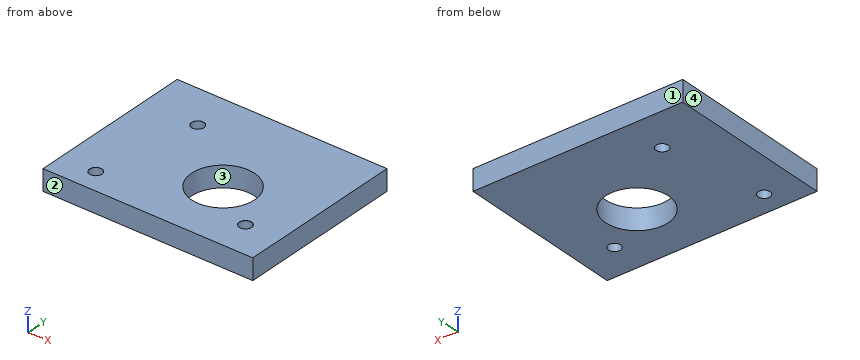
```python
from build123d import *

# Parameters (mm, degrees)
SKETCH1_W                        = 50
SKETCH1_H                        = 40
BOSS_EXTRUDE1_DEPTH              = 2.5
M2_5_CLEARANCE_HOLE2_D           = 2.9
M2_5_CLEARANCE_HOLE2_CSINK_D     = 2.95
M2_5_CLEARANCE_HOLE2_CSINK_ANGLE = 90
SKETCH4_R                        = 7.5
CUT_EXTRUDE1_DEPTH               = 6


with BuildPart() as part:
    # Sketch1 → Boss-Extrude1 (new body, symmetric)
    with BuildSketch(Plane.XY):
        with Locations((16.688846575, 14.654391813)):
            Rectangle(SKETCH1_W, SKETCH1_H)
    extrude(amount=BOSS_EXTRUDE1_DEPTH, both=True)

    # M2.5 Clearance Hole2 (through all)
    with Locations(Plane.XY.offset(2.5)):
        with Locations((4.655068225, 24.562783633), (33.37769315, 2.86), (0, 0)):
            CounterSinkHole(M2_5_CLEARANCE_HOLE2_D / 2, M2_5_CLEARANCE_HOLE2_CSINK_D / 2, counter_sink_angle=M2_5_CLEARANCE_HOLE2_CSINK_ANGLE)

    # Sketch4 → Cut-Extrude1 (cut, through all)
    with BuildSketch(Plane.XY.offset(2.5)):
        with Locations((21.775361697, 10.694915753)):
            Circle(SKETCH4_R)
    extrude(amount=-CUT_EXTRUDE1_DEPTH, mode=Mode.SUBTRACT)


solid = part.part
```
Here's how the part is built. I have some questions about the finished solid (model axes, mm). Face numbers are marked on the shaded views. Round coordinates to 2 decimals unless told otherwise and drop trailing zeros. Write each loop counter-clockwise with the first axis right and the second up, starting at its lowest first coordinate (ties: lowest second). Pieces come first, ordered by that corner, then holes.
Q1. Will this pin go through, and if not, where does the flat tip stop? P1, Ø9, axis at x = 21.78, y = 10.69, coming from the +Z side.
Q2. If we section it at C-C on z = 0.05: Write out the boundary of the cut face in (x, y).
Q3. If we section it at B-B on x = 0: Write out the boundary of the cut face in (y, z) (3 decimals).
Q4. Please list where these lines run through material, in increasing order: probe 1 along X at (y, z) = (2.86, 1.2); probe 2 along X at (y, z) = (0, 1.1); probe 3 along Y at (x, z) = (21.5, 0.45).
Q5. If we mould it in two halves opening along Y, with no side actions, what happens to the marked faces 1, 2, 3 and 4? For each: +Y half, -Y half, draft (parallel to the pull), parting line (faces both ways), or undercut.
Q6. If we section it at D-D on y = 16: Write out the boundary of the cut face in (x, z).
Q7. If we section it at A-A on y = 0: Write out the boundary of the cut face in (x, z) (3 decimals), plus the area to 4 significant figures.
Answer below:
1. P1: passes through
2. outline: (-8.31, -5.35) - (41.69, -5.35) - (41.69, 34.65) - (-8.31, 34.65) - close; hole circle Ø2.9 at (0, 0); hole circle Ø2.9 at (4.66, 24.56); hole circle Ø15 at (21.78, 10.69); hole circle Ø2.9 at (33.38, 2.86)
3. outline: (-5.346, -2.5) - (-1.45, -2.5) - (-1.45, 2.475) - (-1.475, 2.5) - (-5.346, 2.5) - close; (1.45, -2.5) - (34.654, -2.5) - (34.654, 2.5) - (1.475, 2.5) - (1.45, 2.475) - close
4. probe 1: x = -8.31 to 31.93, 34.83 to 41.69
4. probe 2: x = -8.31 to -1.45, 1.45 to 41.69
4. probe 3: y = -5.35 to 3.2, 18.19 to 34.65
5. face 1: +Y half
5. face 2: -Y half
5. face 3: undercut
5. face 4: draft
6. outline: (-8.31, -2.5) - (16.47, -2.5) - (16.47, 2.5) - (-8.31, 2.5) - close; (27.08, -2.5) - (41.69, -2.5) - (41.69, 2.5) - (27.08, 2.5) - close
7. outline: (-8.311, -2.5) - (-1.45, -2.5) - (-1.45, 2.475) - (-1.475, 2.5) - (-8.311, 2.5) - close; (1.45, -2.5) - (41.689, -2.5) - (41.689, 2.5) - (1.475, 2.5) - (1.45, 2.475) - close
7. area: 235.5 mm2
